Source: CAD feature listing. Evaluate the final solid. Frame: model axes, mm. A direction names the side the tool comes from. Give positions to 0.01 mm unless a question says otherwise; leave off trailing zeros. Write each loop counter-clockwise with the first axis right and the second up, starting at its lowest first coordinate (ties: lowest second). Pieces come first, ordered by that corner, then holes. Notation, with made-up numbers: (-1, 39.5) -> (5, 39.5) arc R23 ccw to (5, 54.5) -> close; hole circle Ø9 at (41.25, 11.5). An arc over 180 degrees is marked (long way). Write item = value, one per line.
from build123d import *

# Parameters (mm, degrees)
F1_DEPTH = 170
F2_T     = -0.5


# Not quite as in the source:
# - a feature names something its author has since deleted; it is built from what else it names


with BuildPart() as f1:
    # F0 (on Top) → F1 (new body)
    with BuildSketch(Plane.XY):
        Polygon((16.3101451046, 28.25), (-16.3101451046, 28.25), (-32.6202902092, 0), (-16.3101451046, -28.25), (16.3101451046, -28.25), (32.6202902092, 0), align=None)
    extrude(amount=F1_DEPTH)

    # F2
    f2_openings = [f1.faces().sort_by_distance(p)[0] for p in [
        (0, 0, 170),
    ]]
    offset(amount=F2_T, openings=f2_openings)

    # F3: F1 across face


with BuildPart() as f1_1:
    add(f1.part)
    add(f1.part.mirror(Plane(origin=(-24.032204955, 13.875, 85.25), x_dir=(0.5, 0.8660254038, 0), z_dir=(0.8660254038, -0.5, 0))))

    # F4: F1 across face


with BuildPart() as f1_2:
    add(f1_1.part)
    add(f1_1.part.mirror(Plane(origin=(-24.3208800896, -14.375, 85), x_dir=(0.5, -0.8660254038, 0), z_dir=(-0.8660254038, -0.5, 0))))


solid = f1_2.part
1) Access query for faces 1 (the flat face through (-23.856, 42.319, 83.81)), 2 (the flat face through (23.9, -14.1, 84.1)), 3 (the flat face through (-73.652, 13.569, 83.81)). Directions: +Z, -Z, +X, -X, +Y, -Y. A direction counts if a zero-diameter tool reaches every point of the face in a straight line with its end or side. Return the directions, or none.
Computed:
face_1 = +Z, -Z, +X, +Y
face_2 = +Z
face_3 = +Z, -Z, -X
2) Cut plane C-C (z = 159). State how many separate pieces and enclosed holes the cut face has, then the cut area to 3 significant figures.
Computed:
separate_pieces = 1
enclosed_holes = 5
area = 354 mm²
3) Contact query for flat-ended pins moving along their axis: pin 1 (1.5 mm diameter, centred on x = 3.5, z = 122.5, fed in from -Y); pin 2 (5 mm diameter, centred on x = -33, y = -39.5, fed in from +Z); pin 3 (10 mm diameter, centred on y = -30.5, z = 23, fed in from +X). Output: stop coordinate, or through.
Computed:
pin_1 = -28.25
pin_2 = 0.5
pin_3 = 17.9
4) Cut plane D-D (x = -4). Return the cut outline in (y, z).
Computed:
outline = (-28.25, 0) -> (28.25, 0) -> (28.25, 170) -> (27.75, 170) -> (27.75, 0.5) -> (-27.75, 0.5) -> (-27.75, 170) -> (-28.25, 170) -> close
5) Cut plane A-A (x = -44.5). Return the cut outline in (y, z).
Computed:
outline = (-56.5, 0) -> (56, 0) -> (56, 170) -> (55, 170) -> (55, 0.5) -> (0, 0.5) -> (0, 170) -> (-1, 170) -> (-1, 0.5) -> (-56, 0.5) -> (-56, 170) -> (-56.5, 170) -> close
6) Cut plane B-B (y = -12.5). Return the cut outline in (x, z).
Computed:
outline = (-72.46, 0) -> (25.4, 0) -> (25.4, 170) -> (24.83, 170) -> (24.83, 0.5) -> (-24.83, 0.5) -> (-24.83, 170) -> (-25.98, 170) -> (-25.98, 0.5) -> (-71.88, 0.5) -> (-71.88, 170) -> (-72.46, 170) -> close
7) Material intervals for L1, parallel to Y at x = -61.5, z = 92; L2, parallel to X at y = 21, z = 20.5; L3, parallel to X at y = -23, z = 56, sorted ascending.
Computed:
L1 = -56.5 to -56, -1 to 0, 55 to 56
L2 = -77.94 to -77.36, -76.79 to -76.21, -20.5 to -19.34, 19.92 to 20.5
L3 = -78.52 to -77.94, -19.92 to -18.76, 18.76 to 19.34
8) Draft query along Y for faces 4 (the flat face through (-24.786, 40.931, 84.064)), 5 (the flat face through (-73.22, -14.82, 84.06)), 6 (the flat face through (0, -28.25, 84)), 7 (the flat face through (-32, -1, 170)). Return one class per face: pulls with the +Y half, pulls with the -Y half, needs draft (parallel to the pull), parting line crosses it, or undercut.
Computed:
face_4 = undercut
face_5 = undercut
face_6 = pulls with the -Y half
face_7 = needs draft
